Autodesk Inventor part; units mm, degrees
ref_plane "YZ Plane" through (0, 0, 0) normal (1, 0, 0) x (0, 1, 0)
ref_plane "XZ Plane" through (0, 0, 0) normal (0, 1, 0) x (-1, 0, 0)
ref_plane "XY Plane" through (0, 0, 0) normal (0, 0, 1) x (1, 0, 0)
sketch "Sketch1" plane through (0, 0, 0) normal (0, 1, 0) x (-1, 0, 0)
  line L0 (-15.875, -15.875) -> (15.875, -15.875)
  line L1 (15.875, -15.875) -> (15.875, 15.875)
  line L2 (15.875, 15.875) -> (-15.875, 15.875)
  line L3 (-15.875, 15.875) -> (-15.875, -15.875)
  line L4 (-15.875, -15.875) -> (15.875, 15.875) construction
  line L5 (15.875, -15.875) -> (-15.875, 15.875) construction
  point P0 (0, 0)
  point P1 (0, 0)
  dimension "d0" = 31.75
  dimension "d1" = 31.75
extrude "Extrusion1" add sketch "Sketch1" along normal blind 1.651
hole "Hole1" at (-13.462, 1.651, 13.462) direction (0, -1, 0) diameter 2.159 depth 1.651 tip angle 118 countersink diameter 3.7338 countersink angle 82
hole "Hole2" at (-13.462, 1.651, -13.462) direction (0, -1, 0) diameter 2.159 depth 1.651 tip angle 118 countersink diameter 3.7338 countersink angle 82
hole "Hole3" at (13.462, 1.651, -13.462) direction (0, -1, 0) diameter 2.159 depth 1.651 tip angle 118 countersink diameter 3.7338 countersink angle 82
hole "Hole4" at (13.462, 1.651, 13.462) direction (0, -1, 0) diameter 2.159 depth 1.651 tip angle 118 countersink diameter 3.7338 countersink angle 82
chamfer "Chamfer1" distance 0.0508 angle 45 1 edges at (-13.462, 0, 12.3825)
chamfer "Chamfer2" distance 0.0508 angle 45 1 edges at (13.462, 0, 12.3825)
chamfer "Chamfer3" distance 0.0508 angle 45 1 edges at (13.462, 0, -14.5415)
chamfer "Chamfer4" distance 0.0508 angle 45 1 edges at (-13.462, 0, -14.5415)
properties part number "Housing_Top"
Input: part model. Units: mm. Frame: model coordinates. Round coordinates to 2 decimals unless told otherwise and drop trailing zeros. Answer as CSV lines item,"result". Start each with the question number.
(1) Section A-A, the plane z = 13. State how many separate pieces and enclosed holes the cut face has, plus the area to 3 significant figures.
(2) First-contact query: pin 1 (1.7 mm diameter, centred on x = 13.462, z = 13.462, fed in from -Y); pin 2 (2.5 mm diameter, centred on x = -13.462, z = -13.462, fed in from -Y). Flat tips, straight axial feed; report the tip coordinate or a pass-through.
(3) Draft query along Z for faces 1 (the flat face through (-15.875, 1, 0)), 2 (the cylindrical face through (14.119, 0.393, 12.605)), 3 (the flat face through (0, 1, -15.875)). Return one class per face: released by +Z, released by -Z, zero draft, split by the parting line, or undercut.
(4) Line query: line 1 (Z direction, x = -13.5, y = 0.8) (1 decimal); line 2 (X direction, y = 1.35, z = -12) (3 decimals); line 3 (Z direction, x = 12, y = 1.55) (3 decimals). Output: solid intervals per line, ascending. Write a range as [from, to].
Values found:
1,separate pieces,"3"
1,enclosed holes,"0"
1,area,"44.4 mm²"
2,pin 1,"passes through"
2,pin 2,"stops at y = 0"
3,face 1,"zero draft"
3,face 2,"undercut"
3,face 3,"released by -Z"
4,line 1,"z = [-15.9, -14.6], [-12.3, 12.3], [14.6, 15.9]"
4,line 2,"x = [-15.875, -14.125], [-12.799, 12.799], [14.125, 15.875]"
4,line 3,"z = [-15.875, -14.476], [-12.448, 12.448], [14.476, 15.875]"
